Work out the finished part from the listing and answer in its coordinate system (mm). Face numbers are marked on the shaded views. Coordinates: 2 decimals unless noted, no trailing zeros. Order: outer loops, then holes, each group sorted by start corner. A loop starts at its lowest first (then second) coordinate and runs counter-clockwise, first axis right, second up. Notation, with made-up numbers: (67.25, -15) - (97.25, -15) arc R11 cw to (97.25, 0) - close; hole circle Ø11 at (72, 77). An arc over 180 degrees is marked (long way). Answer as a JSON object with one key per item and string values. Group by question number.
1) Find the intervals of material crossed by line 1 along Y through (x, z) = (0, 2.1); line 2 along X through (y, z) = (-23, 2.3); line 3 along X through (y, z) = (-5, 0.75), in increasing order.
2) Section B-B (y = 0) is taken. Give the vertices of the cut face in (x, z) (1 decimal), plus the area to 3 significant figures.
3) This flat-tipped pin is pushed along its axis until it touches: P1, Ø2.5, axis at x = 0, y = -25.4, coming from the +Z side. Where does it stop, or does it pass through?
4) Section A-A (x = 0) is taken. Give the vertices of the cut face in (y, z) (1 decimal), plus the area to 3 significant figures.
5) Section C-C (z = 2.15) is taken. Give the vertices of the cut face in (x, y) (1 decimal), plus the area to 3 significant figures.
6) The mould has two halves that part along X. Classify the marked faces 1, 2 and 3: released by +X, released by -X, zero draft, split by the parting line, or undercut.
7) Section D-D (y = -12.7) is taken. Give the vertices of the cut face in (x, z) (3 decimals).
from build123d import *

# Parameters (mm, degrees)
SKETCH1_R           = 2.032
BOSS_EXTRUDE1_DEPTH = 3.175


with BuildPart() as part:
    # Sketch1 → Boss-Extrude1 (new body)
    with BuildSketch(Plane.XY):
        with BuildLine():
            Line((2.559372995, 27.959372995), (27.959372995, 2.559372995))
            ThreePointArc((27.959372995, 2.559372995), (29.0195, 0), (27.959372995, -2.559372995))
            Line((27.959372995, -2.559372995), (2.559372995, -27.959372995))
            ThreePointArc((2.559372995, -27.959372995), (-0.442722203, -28.992321993), (-3.104193058, -27.261388113))
            Line((-3.104193058, -27.261388113), (-8.815732721, -17.736388113))
            ThreePointArc((-8.815732721, -17.736388113), (-9.199834878, -16.840700128), (-9.331039662, -15.875))
            Line((-9.331039662, -15.875), (-9.331039662, 15.875))
            ThreePointArc((-9.331039662, 15.875), (-9.199834878, 16.840700128), (-8.815732721, 17.736388113))
            Line((-8.815732721, 17.736388113), (-3.104193058, 27.261388113))
            ThreePointArc((-3.104193058, 27.261388113), (-0.442722203, 28.992321993), (2.559372995, 27.959372995))
        make_face()
        Circle(SKETCH1_R, mode=Mode.SUBTRACT)
        with Locations((0, 25.4)):
            Circle(SKETCH1_R, mode=Mode.SUBTRACT)
        with Locations((0, -25.4)):
            Circle(SKETCH1_R, mode=Mode.SUBTRACT)
        with Locations((25.4, 0)):
            Circle(SKETCH1_R, mode=Mode.SUBTRACT)
        with Locations((0, -12.7)):
            Circle(SKETCH1_R, mode=Mode.SUBTRACT)
    extrude(amount=BOSS_EXTRUDE1_DEPTH)


solid = part.part
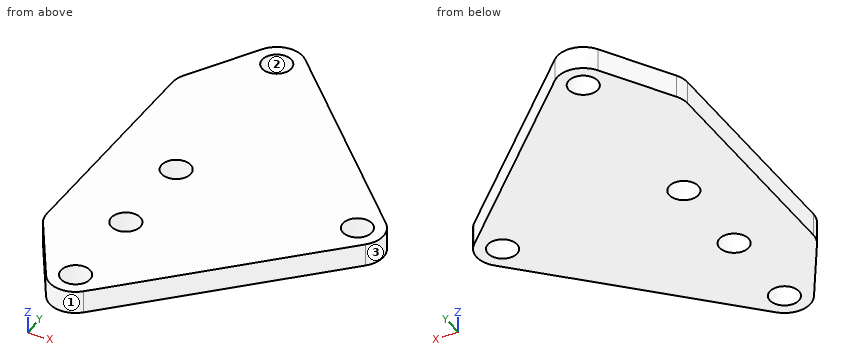
Report:
{
 "1": {"line 1": "y = -29.02 to -27.43, -23.37 to -14.73, -10.67 to -2.03, 2.03 to 23.37, 27.43 to 29.02", "line 2": "x = -5.66 to 7.52", "line 3": "x = -9.33 to 25.52"},
 "2": {"outline": "(-9.3, 0) - (-2, 0) - (-2, 3.2) - (-9.3, 3.2) - close; (2, 0) - (23.4, 0) - (23.4, 3.2) - (2, 3.2) - close; (27.4, 0) - (29, 0) - (29, 3.2) - (27.4, 3.2) - close", "area": "96.0 mm²"},
 "3": {"P1": "passes through"},
 "4": {"outline": "(-29, 0) - (-27.4, 0) - (-27.4, 3.2) - (-29, 3.2) - close; (-23.4, 0) - (-14.7, 0) - (-14.7, 3.2) - (-23.4, 3.2) - close; (-10.7, 0) - (-2, 0) - (-2, 3.2) - (-10.7, 3.2) - close; (2, 0) - (23.4, 0) - (23.4, 3.2) - (2, 3.2) - close; (27.4, 0) - (29, 0) - (29, 3.2) - (27.4, 3.2) - close", "area": "133 mm²"},
 "5": {"outline": "(-9.3, -15.9) arc R3.6 ccw to (-8.8, -17.7) - (-3.1, -27.3) arc R3.6 ccw to (2.6, -28) - (28, -2.6) arc R3.6 ccw to (28, 2.6) - (2.6, 28) arc R3.6 ccw to (-3.1, 27.3) - (-8.8, 17.7) arc R3.6 ccw to (-9.3, 15.9) - close; hole circle Ø4.1 at (0, -25.4); hole circle Ø4.1 at (0, -12.7); hole circle Ø4.1 at (0, 0); hole circle Ø4.1 at (0, 25.4); hole circle Ø4.1 at (25.4, 0)", "area": "1,310 mm²"},
 "6": {"face 1": "split by the parting line", "face 2": "undercut", "face 3": "released by +X"},
 "7": {"outline": "(-9.331, 0) - (-2.032, 0) - (-2.032, 3.175) - (-9.331, 3.175) - close; (2.032, 0) - (17.819, 0) - (17.819, 3.175) - (2.032, 3.175) - close"}
}
